The model under review builds one solid part; all positions refer to its coordinate system, in mm. A direction names the side the tool comes from. Give positions to 0.01 mm unless a question says otherwise; leave off trailing zeros. Order: outer loops, then holes, each group sorted by start corner. A loop starts at its lowest first (then second) coordinate and runs counter-clockwise, first axis right, second up.
```python
from build123d import *

# Parameters (mm, degrees)
SKETCH1_W             = 75
SKETCH1_H             = 15
BOSS_EXTRUDE1_DEPTH   = 15
SKETCH2_W             = 17
SKETCH2_H             = 12.5
CUT_EXTRUDE1_DEPTH    = 12
SKETCH3_W             = 10
SKETCH3_H             = 15
CUT_EXTRUDE2_DEPTH    = 12
F_4_0MM_DOWEL_HOLE2_D = 4
FILLET1_R             = 2


with BuildPart() as part:
    # Sketch1 → Boss-Extrude1 (new body)
    with BuildSketch(Plane(origin=(0, 0, 0), x_dir=(1, 0, 0), z_dir=(0, 1, 0))):
        Rectangle(SKETCH1_W, SKETCH1_H)
    extrude(amount=BOSS_EXTRUDE1_DEPTH)

    # Sketch2 → Cut-Extrude1 (cut)
    with BuildSketch(Plane(origin=(0, 15, 0), x_dir=(1, 0, 0), z_dir=(0, 1, 0))):
        with Locations((-16, -1.25)):
            Rectangle(SKETCH2_W, SKETCH2_H)
        with Locations((16, -1.25)):
            Rectangle(SKETCH2_W, SKETCH2_H)
    extrude(amount=-CUT_EXTRUDE1_DEPTH, mode=Mode.SUBTRACT)

    # Sketch3 → Cut-Extrude2 (cut)
    with BuildSketch(Plane.XZ):
        with Locations((-32.5, 0)):
            Rectangle(SKETCH3_W, SKETCH3_H)
        with Locations((32.5, 0)):
            Rectangle(SKETCH3_W, SKETCH3_H)
        Rectangle(SKETCH3_W, SKETCH3_H)
    extrude(amount=-CUT_EXTRUDE2_DEPTH, mode=Mode.SUBTRACT)

    # Ø4.0mm Dowel Hole2 (through all)
    with Locations(Plane(origin=(0, 12, 0), x_dir=(-1, 0, 0), z_dir=(0, -1, 0))):
        with Locations((32.5, 0), (0, 0), (-32.5, 0)):
            Hole(F_4_0MM_DOWEL_HOLE2_D / 2)

    # Fillet1
    fillet1_edges = [part.edges().sort_by_distance(p)[0] for p in [
        (-37.5, 13.5, -7.5),
        (37.5, 13.5, -7.5),
        (37.5, 13.5, 7.5),
        (-37.5, 13.5, 7.5),
    ]]
    fillet(fillet1_edges, radius=FILLET1_R)


solid = part.part
```
1. Take a section at C-C (z = 0). Count the separate pieces of the cut face and the enclosed holes in it, and give its area (3 significant figures).
2. Take a section at B-B (x = 0). Write out the cut boundary in (y, z).
3. Draft analysis for pull direction Z (two halves, no side actions). For faces 1 (the flat face through (7.5, 9, 1)), 2 (the flat face through (16, 9, -5)), 3 (the cylindrical face through (-30.592, 13.521, -0.601)), state which applies: pulls with the +Z half, pulls with the -Z half, needs draft (parallel to the pull), parting line crosses it, or undercut.
4. For faces 4 (the flat face through (-7.5, 9, 1)), 5 (the flat face through (-1, 12, 2)), 6 (the flat face through (34, 12, 2)), 7 (the flat face through (-31, 12, 2)), list the 3-axis set-ups (+Z, -Z, +X, -X, +Y, -Y) from which the entire face can be reached by the end or side of a thin tool; tool diameter is ignored.
5. Insertion check: pin 1 (5 mm diameter, centred on x = -32.5, z = 0, fed in from -Y); pin 2 (6 mm diameter, centred on x = 16, z = -0.5, fed in from +Y); pin 3 (2.5 mm diameter, centred on x = 0, z = 0, fed in from -Y); pin 4 (6 mm diameter, centred on x = 15, y = 11.5, fed in from +Z). Each pin has a flat end and moves straight along its axis. Give the tip position at first contact, or say it passes through.
6. To check wall thickness, follow line 1 (X direction, y = 10.5, z = 1.25); line 2 (Z direction, x = 32.5, y = 12.75); line 3 (X direction, y = 13, z = -4). State the ranges of each line that lie inside material, in increasing order.
7. Take a section at D-D (y = 14). Write out the cut boundary in (x, z), and give its area (3 significant figures).
8. Take a section at A-A (y = 7.5). Write out the cut boundary in (x, z), and give its area (3 significant figures).
Answer:
1. separate pieces: 4
1. enclosed holes: 0
1. area: 321 mm2
2. outline: (12, -7.5) - (15, -7.5) - (15, -2) - (12, -2) - close; (12, 2) - (15, 2) - (15, 7.5) - (12, 7.5) - close
3. face 1: needs draft
3. face 2: pulls with the +Z half
3. face 3: undercut
4. face 4: +Z, +Y
4. face 5: +Z, -Z, -Y
4. face 6: +Z, -Z, +X, -Y
4. face 7: +Z, -Z, -X, -Y
5. pin 1: stops at y = 12
5. pin 2: stops at y = 3
5. pin 3: passes through
5. pin 4: stops at z = -5
6. line 1: x = -27.5 to -24.5, -7.5 to -5, 5 to 7.5, 24.5 to 27.5
6. line 2: z = -7.5 to -2, 2 to 7.5
6. line 3: x = -37.5 to -24.5, -7.5 to 7.5, 24.5 to 37.5
7. outline: (-37.5, -5.5) arc R2 ccw to (-35.5, -7.5) - (35.5, -7.5) arc R2 ccw to (37.5, -5.5) - (37.5, 5.5) arc R2 ccw to (35.5, 7.5) - (24.5, 7.5) - (24.5, -5) - (7.5, -5) - (7.5, 7.5) - (-7.5, 7.5) - (-7.5, -5) - (-24.5, -5) - (-24.5, 7.5) - (-35.5, 7.5) arc R2 ccw to (-37.5, 5.5) - close; hole circle Ø4 at (-32.5, 0); hole circle Ø4 at (0, 0); hole circle Ø4 at (32.5, 0)
7. area: 659 mm2
8. outline: (-27.5, -7.5) - (-5, -7.5) - (-5, 7.5) - (-7.5, 7.5) - (-7.5, -5) - (-24.5, -5) - (-24.5, 7.5) - (-27.5, 7.5) - close; (5, -7.5) - (27.5, -7.5) - (27.5, 7.5) - (24.5, 7.5) - (24.5, -5) - (7.5, -5) - (7.5, 7.5) - (5, 7.5) - close
8. area: 250 mm2
